Answer from the drawing. Dimensions are ordinates in mm from the lowest x, y and z of the part. A direction names the side the tool comes from. Round coordinates to 2 decimals unless told otherwise and drop trailing zeros. Loops run counter-clockwise (first coordinate to the right, second up) from the corner with the lowest first, then second, coordinate; pieces in that order, holes last. Notation, with made-up numbers: M 11,2.5 L 51,2.5 A35 ccw 51,35.5 Z; hole C 35.25,80.5 d11. An arc over 180 degrees is marked long. Answer as a JSON object with one key per item and string values.
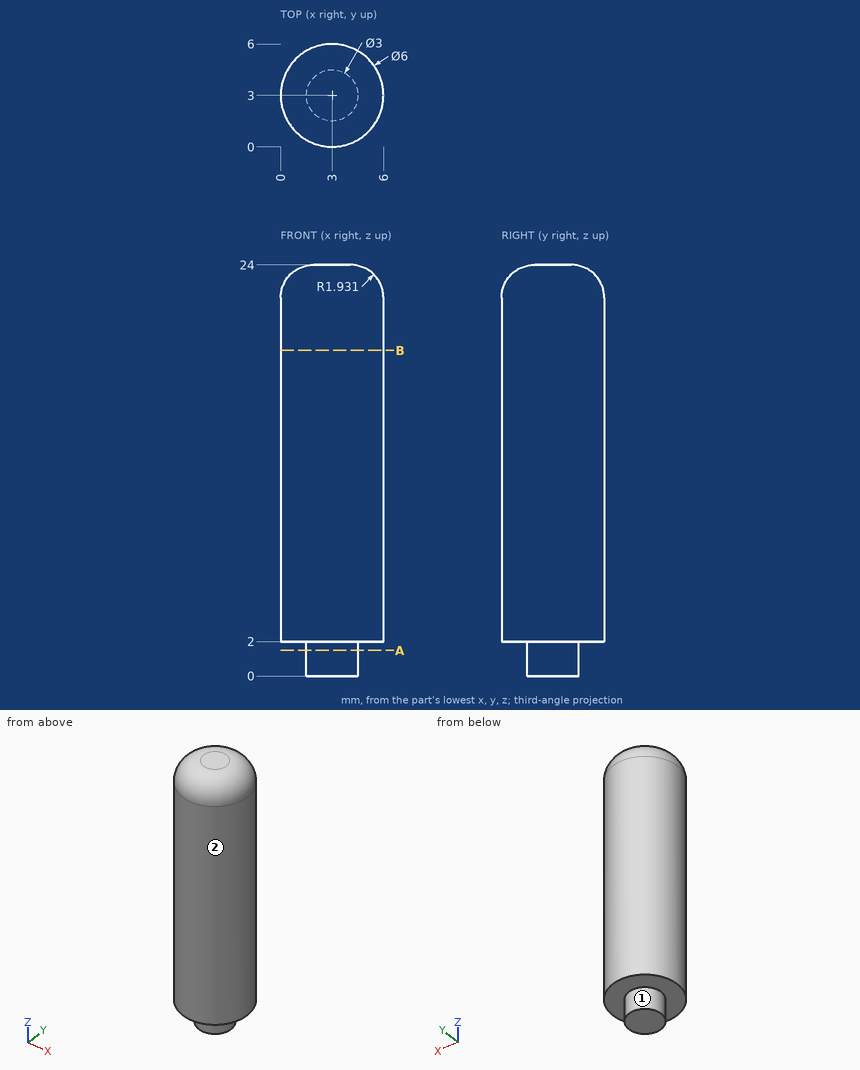
Item 1: Which of the six approach directions +Z, -Z, +X, -X, +Y, -Y give full straight-line access (tool end or side, diameter ignored) to the marked faces 1 and 2?
Values follow:
{"face 1": "-Z", "face 2": "+Z, -Z"}
Item 2: The part is cut by section A-A (z = 1.5). Give the vertices of the cut face in (x, y).
Values follow:
{"outline": "C 3,3 d3"}
Item 3: Straight lines are drawn through the part: line 1 (Y direction, x = 2.65, z = 6.25); line 2 (X direction, y = 0.85, z = 15.25); line 3 (X direction, y = 5, z = 19.25) (1 decimal). For each, find the intervals that lie inside material, in ascending order.
Values follow:
{"line 1": "0.02 to 5.98", "line 2": "0.91 to 5.09", "line 3": "0.8 to 5.2"}
Item 4: Flat-ended cylindrical pins translate along their axes: P1, Ø3, axis at x = 2.5, z = 10, coming from the -Y side; P2, Ø1.5, axis at x = 4.5, z = 11, coming from the -Y side (1 decimal); P3, Ø1, axis at x = 1, y = 3, coming from the +Z side. Find the tip coordinate at first contact, or state that the pin passes through.
Values follow:
{"P1": "y = 0", "P2": "y = 0.1", "P3": "z = 23.95"}
Item 5: The part is cut by section B-B (z = 19). Give the vertices of the cut face in (x, y), then the cut area to 3 significant figures.
Values follow:
{"outline": "C 3,3 d6", "area": "28.3 mm^2"}
